```python
from build123d import *

# Parameters (mm, degrees)
SKETCH4_R                         = 2.413
CUT_EXTRUDE1_DEPTH                = 94.3255592
CIRPATTERN1_COUNT                 = 8
CUT_EXTRUDE7_START                = -4.826
SKETCH18_R                        = 63.5
SKETCH18_R_2                      = 2.413
CUT_EXTRUDE7_DEPTH                = 4.826
SKETCH17_R                        = 33.02
CUT_EXTRUDE6_DEPTH                = 7.112
PIPE_TAP_DRILL_FOR_3_8_TAP1_D     = 14.2748
PIPE_TAP_DRILL_FOR_3_8_TAP1_DEPTH = 12.7
PIPE_TAP_DRILL_FOR_3_8_TAP1_TIP   = 4.288582582
F_3_8_0_375_DIAMETER_HOLE1_D      = 9.525
F_3_8_0_375_DIAMETER_HOLE1_DEPTH  = 63.5
F_3_8_0_375_DIAMETER_HOLE1_TIP    = 2.861598698
SKETCH19_R                        = 50.8
SKETCH19_R_2                      = 46.0248
SEAL_GROOVE_DEPTH                 = 3.1369


with BuildPart() as part:
    # Sketch16 → Revolve1 (revolve)
    with BuildSketch(Plane(origin=(0, 0, 0), x_dir=(1, 0, 0), z_dir=(0, 1, 0)), mode=Mode.PRIVATE) as revolve1_sk:
        Polygon((7.9375, -25.4), (63.5, -25.4), (63.5, 0), (14.2875, 0), (14.2875, -16.66875), (11.176, -16.66875), (11.176, -23.8125), (7.9375, -23.8125), align=None)
    revolve(revolve1_sk.sketch.rotate(Axis((0, 0, 0), (0, 0, 1)), 180), axis=Axis((0, 0, 0), (0, 0, 1)))

    # Sketch4 → Cut-Extrude1 (cut, through all)
    with BuildSketch(Plane.XY.offset(25.4)):
        with Locations((52.799715283, -21.87035816)):
            Circle(SKETCH4_R)
    cut_extrude1 = extrude(amount=-CUT_EXTRUDE1_DEPTH, mode=Mode.SUBTRACT)

    # CirPattern1: Cut-Extrude1 ×8 about axis
    cirpattern1_axis = Axis((0, 0, 0), (0, 0, 1))
    for i in range(1, CIRPATTERN1_COUNT):
        add(cut_extrude1.rotate(cirpattern1_axis, i * 360 / CIRPATTERN1_COUNT), mode=Mode.SUBTRACT)

    # Sketch18 → Cut-Extrude7 (cut)
    with BuildSketch(Plane(origin=(0, 0, 0), x_dir=(-1, 0, 0), z_dir=(0, 0, -1)).offset(CUT_EXTRUDE7_START)):
        Circle(SKETCH18_R)
        with Locations(Location((-21.87035816, -52.799715283, 0), (0, 0, 225))):
            Circle(SKETCH18_R_2, mode=Mode.SUBTRACT)
        with Locations(Location((-52.799715283, -21.87035816, 0), (0, 0, 180))):
            Circle(SKETCH18_R_2, mode=Mode.SUBTRACT)
        with Locations(Location((21.87035816, -52.799715283, 0), (0, 0, 270))):
            Circle(SKETCH18_R_2, mode=Mode.SUBTRACT)
        with Locations(Location((52.799715283, -21.87035816, 0), (0, 0, 315))):
            Circle(SKETCH18_R_2, mode=Mode.SUBTRACT)
        with Locations((-52.799715283, 21.87035816)):
            Circle(SKETCH18_R_2, mode=Mode.SUBTRACT)
        with BuildLine():
            Line((-38.437855153, -3.307865299), (-41.774591166, -3.307865299))
            ThreePointArc((-41.774591166, -3.307865299), (-44.06614875, -2.330452348), (-44.946809919, 0))
            add(Edge.make_bspline(
                [(-33.928933872, -7.134607515), (-33.928385732, -7.137933992), (-33.833010931, -7.716207568), (-33.613407498, -8.8658869), (-33.198558281, -10.568668335), (-32.697590483, -12.252202478), (-32.111368753, -13.912132646), (-31.440982434, -15.544140087), (-30.6877424, -17.143955629), (-29.853178348, -18.707371069), (-28.939035433, -20.230250424), (-27.947270591, -21.708540989), (-26.880048317, -23.138284208), (-25.739735978, -24.515626324), (-24.52889861, -25.836828804), (-23.250293206, -27.098278486), (-21.906862513, -28.296497465), (-20.501728328, -29.428152646), (-19.038184319, -30.490064988), (-17.519688378, -31.479218369), (-15.949854523, -32.392768086), (-14.332444364, -33.228048947), (-12.67135816, -33.982582934), (-10.970625473, -34.654086422), (-9.23439546, -35.240476937), (-7.466926803, -35.739879413), (-5.672577322, -36.150631964), (-3.855793286, -36.471291116), (-2.021098439, -36.700636517), (-0.173082793, -36.837675086), (1.683608814, -36.881644605), (3.544288344, -36.832016725), (5.404236353, -36.688499397), (7.258713917, -36.451038699), (9.102974666, -36.119820063), (10.932276886, -35.695268896), (12.741895669, -35.178050585), (14.527135072, -34.569069886), (16.283340262, -33.869469699), (18.005909603, -33.080629222), (19.690306669, -32.204161496), (21.332072136, -31.241910334), (22.926835541, -30.195946649), (24.470326852, -29.068564177), (25.958387849, -27.862274615), (27.386983251, -26.579802172), (28.752211598, -25.224077558), (30.05031582, -23.798231409), (31.277693495, -22.305587173), (32.430906752, -20.749653473), (33.506691795, -19.134115953), (34.501968029, -17.462828639), (35.41384675, -15.739804832), (36.239639383, -13.969207544), (36.976865247, -12.155339516), (37.623258819, -10.302632827), (38.176776478, -8.415638129), (38.635602708, -6.499013531), (38.99815575, -4.557513153), (39.263092672, -2.595975388), (39.429313851, -0.619310898), (39.495966855, 1.367509636), (39.462449705, 3.359467962), (39.328413504, 5.351510889), (39.09376444, 7.338563062), (38.758665131, 9.315539846), (38.323535331, 11.277360294), (37.789051968, 13.218960162), (37.15614853, 15.135304935), (36.426013787, 17.021402835), (35.600089858, 18.872317778), (34.680069611, 20.683182241), (33.667893419, 22.449210007), (32.565745258, 24.165708766), (31.376048171, 25.828092515), (30.101459097, 27.431893755), (28.744863072, 28.972775422), (27.309366835, 30.446542545), (25.798291819, 31.849153584), (24.215166578, 33.176731426), (22.563718643, 34.425574005), (20.847865831, 35.59216452), (19.071707037, 36.673181218), (17.239512511, 37.665506723), (15.355713667, 38.566236878), (13.424892429, 39.37268908), (11.451770141, 40.082410076), (9.441196087, 40.693183217), (7.398135616, 41.203035118), (5.327657937, 41.610241741), (3.234923583, 41.913333848), (1.125171597, 42.11110184), (-0.996293545, 42.202599933), (-3.124115223, 42.187149688), (-5.252898166, 42.06434287), (-7.377222085, 41.834043617), (-9.491655438, 41.49638993), (-11.590769276, 41.051794458), (-13.669151145, 40.500944594), (-15.721418994, 39.844801852), (-17.742235078, 39.084600556), (-19.726319787, 38.221845804), (-21.668465399, 37.258310751), (-23.563549696, 36.196033176), (-25.406549423, 35.037311368), (-27.192553543, 33.784699317), (-28.916776264, 32.441001244), (-30.574569796, 31.009265451), (-32.161436808, 29.492777532), (-33.673042551, 27.895052942), (-35.10522661, 26.219828948), (-36.454014261, 24.471055979), (-37.715627401, 22.652888394), (-38.88649501, 20.769674689), (-39.963263134, 18.825947167), (-40.942804349, 16.826411093), (-41.822226678, 14.775933368), (-42.59888195, 12.679530733), (-43.27037356, 10.54235755), (-43.834563622, 8.369693173), (-44.289579482, 6.166928958), (-44.619434592, 4.032631678), (-44.788721316, 2.443473873), (-44.861866668, 1.505376084), (-44.887603288, 1.129504244), (-44.905146434, 0.847378207), (-44.920882878, 0.565074904), (-44.934972992, 0.282611952), (-44.942863945, 0.09421189), (-44.946809919, 0)],
                knots=[0.028816302, 0.028816302, 0.028816302, 0.028816302, 0.028857006, 0.035892384, 0.042943403, 0.050010121, 0.057092589, 0.064190856, 0.07130497, 0.078434976, 0.085580915, 0.092742831, 0.099920762, 0.107114747, 0.114324823, 0.121551027, 0.128793394, 0.136051958, 0.143326753, 0.150617811, 0.157925165, 0.165248846, 0.172588885, 0.179945312, 0.187318157, 0.194707448, 0.202113215, 0.209535486, 0.216974287, 0.224429648, 0.231901594, 0.239390153, 0.246895349, 0.25441721, 0.261955761, 0.269511026, 0.277083032, 0.284671801, 0.29227736, 0.299899731, 0.307538938, 0.315195006, 0.322867957, 0.330557814, 0.338264601, 0.345988339, 0.353729051, 0.36148676, 0.369261487, 0.377053255, 0.384862084, 0.392687996, 0.400531013, 0.408391155, 0.416268443, 0.424162899, 0.432074542, 0.440003393, 0.447949473, 0.455912802, 0.463893399, 0.471891284, 0.479906477, 0.487938998, 0.495988866, 0.5040561, 0.51214072, 0.520242745, 0.528362193, 0.536499083, 0.544653435, 0.552825266, 0.561014596, 0.569221442, 0.577445824, 0.585687758, 0.593947263, 0.602224358, 0.61051906, 0.618831386, 0.627161355, 0.635508984, 0.643874291, 0.652257292, 0.660658007, 0.66907645, 0.677512641, 0.685966595, 0.69443833, 0.702927863, 0.711435211, 0.71996039, 0.728503417, 0.737064309, 0.745643082, 0.754239753, 0.762854337, 0.771486853, 0.780137315, 0.788805739, 0.797492143, 0.806196542, 0.814918952, 0.823659389, 0.832417868, 0.841194407, 0.849989019, 0.858801722, 0.86763253, 0.87648146, 0.885348526, 0.894233744, 0.90313713, 0.912058699, 0.920998466, 0.929956446, 0.938932655, 0.947927107, 0.956939818, 0.965970803, 0.975020076, 0.984087653, 0.992036809, 0.994310574, 0.995447886, 0.996585485, 0.99772337, 0.998861542, 1, 1, 1, 1], degree=3))
            ThreePointArc((-33.928933872, -7.134607515), (-35.480900338, -4.393511216), (-38.437855153, -3.307865299))
        make_face(mode=Mode.SUBTRACT)
        with Locations((-21.87035816, 52.799715283)):
            Circle(SKETCH18_R_2, mode=Mode.SUBTRACT)
        with Locations((52.799715283, 21.87035816)):
            Circle(SKETCH18_R_2, mode=Mode.SUBTRACT)
        with Locations(Location((21.87035816, 52.799715283, 0), (0, 0, 45))):
            Circle(SKETCH18_R_2, mode=Mode.SUBTRACT)
    extrude(amount=CUT_EXTRUDE7_DEPTH, mode=Mode.SUBTRACT)

    # Sketch17 → Cut-Extrude6 (cut)
    with BuildSketch(Plane(origin=(0, 0, 0), x_dir=(-1, 0, 0), z_dir=(0, 0, -1))):
        Circle(SKETCH17_R)
    extrude(amount=-CUT_EXTRUDE6_DEPTH, mode=Mode.SUBTRACT)

    # Pipe Tap Drill for 3/8 Tap1
    with Locations(Plane(origin=(-63.5, 0, 13.55725), x_dir=(0, 0, -1), z_dir=(-1, 0, 0))):
        with Locations((0, 0)):
            Hole(PIPE_TAP_DRILL_FOR_3_8_TAP1_D / 2, depth=PIPE_TAP_DRILL_FOR_3_8_TAP1_DEPTH)
            with Locations((0, 0, -(PIPE_TAP_DRILL_FOR_3_8_TAP1_DEPTH + PIPE_TAP_DRILL_FOR_3_8_TAP1_TIP / 2))):  # 118° drill point
                Cone(0, PIPE_TAP_DRILL_FOR_3_8_TAP1_D / 2, PIPE_TAP_DRILL_FOR_3_8_TAP1_TIP, mode=Mode.SUBTRACT)

    # 3/8 (0.375) Diameter Hole1
    with Locations(Plane.ZY.offset(63.5)):
        with Locations((13.55725, 0)):
            Hole(F_3_8_0_375_DIAMETER_HOLE1_D / 2, depth=F_3_8_0_375_DIAMETER_HOLE1_DEPTH)
            with Locations((0, 0, -(F_3_8_0_375_DIAMETER_HOLE1_DEPTH + F_3_8_0_375_DIAMETER_HOLE1_TIP / 2))):  # 118° drill point
                Cone(0, F_3_8_0_375_DIAMETER_HOLE1_D / 2, F_3_8_0_375_DIAMETER_HOLE1_TIP, mode=Mode.SUBTRACT)

    # Sketch19 → Seal Groove (cut)
    with BuildSketch(Plane(origin=(0, 0, 4.826), x_dir=(-1, 0, 0), z_dir=(0, 0, -1))):
        Circle(SKETCH19_R)
        Circle(SKETCH19_R_2, mode=Mode.SUBTRACT)
    extrude(amount=-SEAL_GROOVE_DEPTH, mode=Mode.SUBTRACT)


solid = part.part
```
CAD build for the part. Positions are in the model's coordinates, mm. A direction names the side the tool comes from. Round coordinates to 2 decimals unless told otherwise and drop trailing zeros.
Item 1: Drop flat-ended pins along their axis: pin 1 Ø1 at (y, z) = (41.5, 14.5) entering from -X; pin 2 Ø10 at (x, z) = (10.5, 11.5) entering from -Y; pin 3 Ø1.7 at (x, z) = (40.5, 1.5) entering from -Y; pin 4 Ø4 at (x, y) = (21.87, 52.8) entering from +Z. Give the stop position or say it passes through.
Filled in:
pin 1: stops at x = -48.49
pin 2: stops at y = -63.26
pin 3: stops at y = -3.31
pin 4: passes through
Item 2: Mould opens along Y. For faces 4 (the flat face through (9, 7, 16.669)), 5 (the flat face through (40, -3.308, 2)), 6 (the flat face through (-1, 13, 25.4)) say: released by +Y, released by -Y, zero draft, split by the parting line, or undercut.
Filled in:
face 4: undercut
face 5: released by -Y
face 6: zero draft
Item 3: Tool access for faces 1 (the cylindrical face through (-31.5, 9.9, 3.5)), 2 (the cylindrical face through (-57.06, 2.73, 20.15)), 3 (the cylindrical face through (21.146, 55.101, 15.257)): list every direction of +Z, -Z, +X, -X, +Y, -Y with a clear straight run to the whole face (end or side of a thin tool).
Filled in:
face 1: -Z
face 2: -X
face 3: +Z, -Z
Item 4: Drill centre lines: L1, parallel to Y at x = 28, z = 7.25; L2, parallel to Y at x = 6, z = 7; L3, parallel to Y at x = 0, z = 10.75. Where is each one in solid material? Low to high.
Filled in:
L1: y = -56.99 to -42.39, -36.53 to 36.53, 42.39 to 56.99
L2: y = -63.22 to -50.44, -45.63 to -32.47, 32.47 to 45.63, 50.44 to 63.22
L3: y = -63.5 to -14.29, 14.29 to 63.5
